Check sheet for the drawn part. Datum: minimum x, y, z corner. Units: mm. A direction names the side the tool comes from. Round coordinates to 2 decimals unless told otherwise and drop trailing zeros. Answer as a JSON object with one key per item and string values. Group by question number.
1) Set-up check for the marked faces 4 and 5: record each of +Z, -Z, +X, -X, +Y, -Y from which the full face is reachable in a straight line by a thin tool's end or side.
2) Mould release check, pull along X, two halves, no side actions. Record for the marked faces 1, 2 and 3: +X half, -X half, draft (parallel to the pull), parting line (faces both ways), or undercut.
3) Thickness scan on line 1 (X direction, y = 14, z = 3) (1 decimal); line 2 (Z direction, x = 2, y = 7.25) (1 decimal). Record the ranges inside material, lowest first.
4) Go/stop test with a flat-tipped pin: pin 1 Ø3 at (x, y) = (3.5, 7) entering from +Z. Record where the tip stops, or that it passes through.
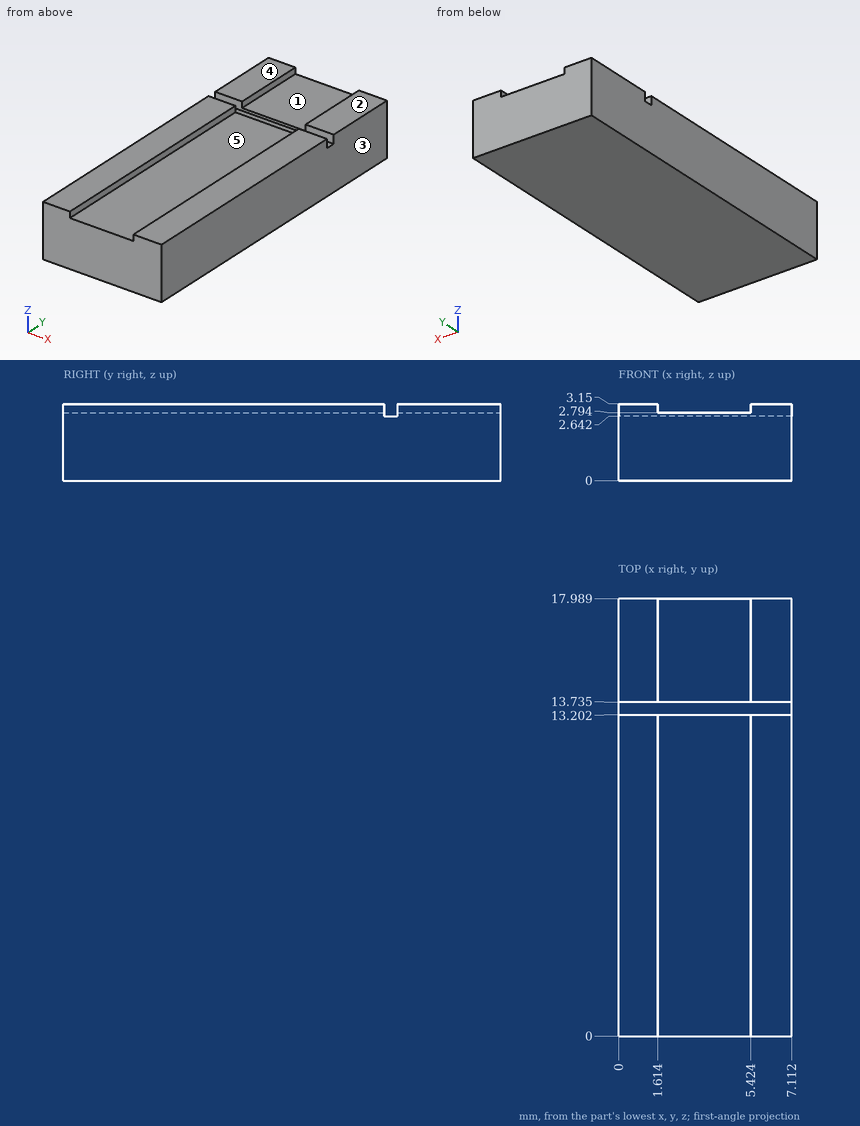
Returned:
{
 "1": {"face 4": "+Z, +X, -X, +Y, -Y", "face 5": "+Z, +Y, -Y"},
 "2": {"face 1": "undercut", "face 2": "draft", "face 3": "+X half"},
 "3": {"line 1": "0 to 1.6, 5.4 to 7.1", "line 2": "0 to 2.8"},
 "4": {"pin 1": "z = 2.79"}
}
